Geometry check sheet. Reference: the model listing, model coordinates, mm. A direction names the side the tool comes from. Round coordinates to 2 decimals unless told otherwise and drop trailing zeros. Order: outer loops, then holes, each group sorted by start corner. A loop starts at its lowest first (then second) coordinate and runs counter-clockwise, first axis right, second up.
(1) Cross-section at B-B on x = 50. Enter the section's corners in (y, z) (3 decimals), and give its area (3 significant figures).
(2) Set-up check for faces 1 (the face through (-1, 42, -55)), 2 (the face through (-66.869, 8.351, -77.185)), 3 (the face through (64.545, 49, -44)): record each of +Z, -Z, +X, -X, +Y, -Y from which the full face is reachable in a straight line by a thin tool's end or side.
(3) Cross-section at C-C on y = 30. Enter the section's corners in (x, z) (3 decimals).
(4) Thickness scan on L1, parallel to Z at x = -39, y = 37 (3 decimals); L2, parallel to X at y = 35.5, z = -9.5 (3 decimals); L3, parallel to Y at x = -33.5, z = -15.5 (3 decimals). Record the ranges inside material, lowest first.
(5) Gauge pin test, flat ends, axial feed: P1, Ø1, axis at y = -34, z = -53.5, coming from the +X side; P2, Ø5, axis at y = 29, z = -65.5, coming from the +X side; P3, Ø6, axis at y = -37.5, z = -73.5, coming from the -X side; P4, Ø10.5, axis at x = -25.5, y = 41.5, coming from the -Z side. Record the tip position at first contact, or that the pin passes through.
(6) Draft check along Y on faces 4 (the face through (-1, 1, 0)), 5 (the face through (-1, 48.755, -28)), 6 (the face through (-1, 50, -27)). Enter one of: pulls with the +Y half, pulls with the -Y half, needs draft (parallel to the pull), parting line crosses it, or undercut.
(7) Cross-section at D-D on y = -15.5. Enter the section's corners in (x, z) (3 decimals), and give its area (3 significant figures).
(8) Cross-section at A-A on z = -29.5. Enter the section's corners in (x, y) (3 decimals), and give its area (3 significant figures).
from build123d import *

# Parameters (mm, degrees)
SKETCH1_W                      = 155
SKETCH1_H                      = 100
BASE_FLANGE2_DEPTH             = 1.245
EDGE_FLANGE3_STRIP_W           = 8.4
EDGE_FLANGE3_STRIP_H           = 1.245
EDGE_FLANGE3_STRIP_CUT_DEPTH   = 155
EDGE_FLANGE3_DEPTH             = 155
CUT_EXTRUDE2_START             = -1.245
CUT_EXTRUDE2_OUTLINE_W         = 10
CUT_EXTRUDE2_OUTLINE_H         = 102
CUT_EXTRUDE2_DEPTH             = 2.955
EDGE_FLANGE4_STRIP_W           = 8.4
EDGE_FLANGE4_STRIP_H           = 1.245
EDGE_FLANGE4_STRIP_CUT_DEPTH   = 97.045
EDGE_FLANGE4_STRIP_2_W         = 8.4
EDGE_FLANGE4_STRIP_2_H         = 1.245
EDGE_FLANGE4_STRIP_CUT_2_DEPTH = 97.045
EDGE_FLANGE4_DEPTH             = 97.045
EDGE_FLANGE4_BEND_DEPTH        = 97.045
EDGE_FLANGE5_STRIP_W           = 8.4
EDGE_FLANGE5_STRIP_H           = 1.245
EDGE_FLANGE5_STRIP_CUT_DEPTH   = 129.09
EDGE_FLANGE5_DEPTH             = 129.09
CUT_EXTRUDE3_DEPTH             = 192.224057064
EDGE_FLANGE6_STRIP_W           = 8.4
EDGE_FLANGE6_STRIP_H           = 1.245
EDGE_FLANGE6_STRIP_CUT_DEPTH   = 129.09
EDGE_FLANGE6_DEPTH             = 129.09
EDGE_FLANGE7_START             = -64.545
EDGE_FLANGE7_DEPTH             = 129.09
EDGE_FLANGE7_2_DEPTH           = 129.09


# Read off the part's stored shape, not the designer's step: Cut-Extrude2, Edge-Flange7
# Sheet-metal steps are written as plain solids
with BuildPart() as part:
    # Sketch1 → Base-Flange2 (new body)
    with BuildSketch(Plane.XY):
        Rectangle(SKETCH1_W, SKETCH1_H)
    extrude(amount=-BASE_FLANGE2_DEPTH)

    # Edge-Flange3 strip (across the edge) → Edge-Flange3 strip cut (cut)
    with BuildSketch(Plane(origin=(77.5, -50, -1.245), x_dir=(0, 1, 0), z_dir=(-1, 0, 0))):
        with Locations((-1.245, -0.6225)):
            Rectangle(EDGE_FLANGE3_STRIP_W, EDGE_FLANGE3_STRIP_H)
    extrude(amount=EDGE_FLANGE3_STRIP_CUT_DEPTH, mode=Mode.SUBTRACT)

    # Edge-Flange3 section (across the edge) → Edge-Flange3 (add)
    with BuildSketch(Plane(origin=(77.5, -50, -1.245), x_dir=(0, 1, 0), z_dir=(-1, 0, 0))):
        with BuildLine():
            Line((0, 1.71), (0, 112.955))
            Line((0, 112.955), (1.245, 112.955))
            Line((1.245, 112.955), (1.245, 1.71))
            ThreePointArc((1.245, 1.71), (1.745847404, 0.500847404), (2.955, 0))
            Line((2.955, 0), (2.955, -1.245))
            ThreePointArc((2.955, -1.245), (0.865499462, -0.379500538), (0, 1.71))
        make_face()
    extrude(amount=EDGE_FLANGE3_DEPTH)

    # Cut-Extrude2 outline → Cut-Extrude2 (cut)
    with BuildSketch(Plane(origin=(0, 0, -1.245), x_dir=(-1, 0, 0), z_dir=(0, 0, -1)).offset(CUT_EXTRUDE2_START)):
        with Locations((72.5, 0)):
            Rectangle(CUT_EXTRUDE2_OUTLINE_W, CUT_EXTRUDE2_OUTLINE_H)
        with Locations((-72.5, 0)):
            Rectangle(CUT_EXTRUDE2_OUTLINE_W, CUT_EXTRUDE2_OUTLINE_H)
    extrude(amount=CUT_EXTRUDE2_DEPTH, mode=Mode.SUBTRACT)

    # Edge-Flange4 strip (across the edge) → Edge-Flange4 strip cut (cut)
    with BuildSketch(Plane(origin=(67.5, 50, -1.245), x_dir=(-1, 0, 0), z_dir=(0, -1, 0))):
        with Locations((-1.245, -0.6225)):
            Rectangle(EDGE_FLANGE4_STRIP_W, EDGE_FLANGE4_STRIP_H)
    extrude(amount=EDGE_FLANGE4_STRIP_CUT_DEPTH, mode=Mode.SUBTRACT)

    # Edge-Flange4 strip 2 (across the edge) → Edge-Flange4 strip cut 2 (cut)
    with BuildSketch(Plane(origin=(-67.5, -47.045, -1.245), x_dir=(1, 0, 0), z_dir=(0, 1, 0))):
        with Locations((-1.245, -0.6225)):
            Rectangle(EDGE_FLANGE4_STRIP_2_W, EDGE_FLANGE4_STRIP_2_H)
    extrude(amount=EDGE_FLANGE4_STRIP_CUT_2_DEPTH, mode=Mode.SUBTRACT)

    # Edge-Flange4 section (across the edge) → Edge-Flange4 (add)
    with BuildSketch(Plane(origin=(67.5, 50, -1.245), x_dir=(-1, 0, 0), z_dir=(0, -1, 0))):
        with BuildLine():
            Line((0, 1.71), (0, 98.755))
            Line((0, 98.755), (1.245, 98.755))
            Line((1.245, 98.755), (1.245, 1.71))
            ThreePointArc((1.245, 1.71), (1.745847404, 0.500847404), (2.955, 0))
            Line((2.955, 0), (2.955, -1.245))
            ThreePointArc((2.955, -1.245), (0.865499462, -0.379500538), (0, 1.71))
        make_face()
    extrude(amount=EDGE_FLANGE4_DEPTH)

    # Edge-Flange4 section 2 (across the edge) → Edge-Flange4 bend (add)
    with BuildSketch(Plane(origin=(-67.5, -47.045, -1.245), x_dir=(1, 0, 0), z_dir=(0, 1, 0))):
        with BuildLine():
            Line((0, 1.71), (0, 98.755))
            Line((0, 98.755), (1.245, 98.755))
            Line((1.245, 98.755), (1.245, 1.71))
            ThreePointArc((1.245, 1.71), (1.745847404, 0.500847404), (2.955, 0))
            Line((2.955, 0), (2.955, -1.245))
            ThreePointArc((2.955, -1.245), (0.865499462, -0.379500538), (0, 1.71))
        make_face()
    extrude(amount=EDGE_FLANGE4_BEND_DEPTH)

    # Edge-Flange5 strip (across the edge) → Edge-Flange5 strip cut (cut)
    with BuildSketch(Plane(origin=(-64.545, 50, -1.245), x_dir=(0, -1, 0), z_dir=(1, 0, 0))):
        with Locations((-1.245, -0.6225)):
            Rectangle(EDGE_FLANGE5_STRIP_W, EDGE_FLANGE5_STRIP_H)
    extrude(amount=EDGE_FLANGE5_STRIP_CUT_DEPTH, mode=Mode.SUBTRACT)

    # Edge-Flange5 section (across the edge) → Edge-Flange5 (add)
    with BuildSketch(Plane(origin=(-64.545, 50, -1.245), x_dir=(0, -1, 0), z_dir=(1, 0, 0))):
        with BuildLine():
            Line((0, 1.71), (0, 53.755))
            Line((0, 53.755), (1.245, 53.755))
            Line((1.245, 53.755), (1.245, 1.71))
            ThreePointArc((1.245, 1.71), (1.745847404, 0.500847404), (2.955, 0))
            Line((2.955, 0), (2.955, -1.245))
            ThreePointArc((2.955, -1.245), (0.865499462, -0.379500538), (0, 1.71))
        make_face()
    extrude(amount=EDGE_FLANGE5_DEPTH)

    # Sketch26 → Cut-Extrude3 (cut, through all)
    with BuildSketch(Plane(origin=(67.5, 0, 0), x_dir=(0, 0, -1), z_dir=(1, 0, 0))):
        Polygon((55, 50), (55, 34.789940387), (100, -18.83897128), (100, 50), align=None)
    extrude(amount=-CUT_EXTRUDE3_DEPTH, mode=Mode.SUBTRACT)

    # Edge-Flange6 strip (across the edge) → Edge-Flange6 strip cut (cut)
    with BuildSketch(Plane(origin=(-64.545, 48.755, -55), x_dir=(0, 0, 1), z_dir=(1, 0, 0))):
        with Locations((-1.245, -0.6225)):
            Rectangle(EDGE_FLANGE6_STRIP_W, EDGE_FLANGE6_STRIP_H)
    extrude(amount=EDGE_FLANGE6_STRIP_CUT_DEPTH, mode=Mode.SUBTRACT)

    # Edge-Flange6 section (across the edge) → Edge-Flange6 (add)
    with BuildSketch(Plane(origin=(-64.545, 48.755, -55), x_dir=(0, 0, 1), z_dir=(1, 0, 0))):
        with BuildLine():
            Line((0, 1.71), (0, 13.965059613))
            Line((0, 13.965059613), (1.245, 13.965059613))
            Line((1.245, 13.965059613), (1.245, 1.71))
            ThreePointArc((1.245, 1.71), (1.745847404, 0.500847404), (2.955, 0))
            Line((2.955, 0), (2.955, -1.245))
            ThreePointArc((2.955, -1.245), (0.865499462, -0.379500538), (0, 1.71))
        make_face()
    extrude(amount=EDGE_FLANGE6_DEPTH)

    # Edge-Flange7 outline → Edge-Flange7 (cut)
    with BuildSketch(Plane.YZ.offset(EDGE_FLANGE7_START)):
        with BuildLine():
            Line((34.789940387, -55), (35.449768265, -54.446338671))
            ThreePointArc((35.449768265, -54.446338671), (36.338536128, -53.933208306), (37.349205652, -53.755))
            Line((37.349205652, -53.755), (34.789940387, -53.755))
            Line((34.789940387, -53.755), (34.789940387, -55))
        make_face()
    extrude(amount=EDGE_FLANGE7_DEPTH, mode=Mode.SUBTRACT)

    # Edge-Flange7 2 outline → Edge-Flange7 2 (add)
    with BuildSketch(Plane.YZ.offset(EDGE_FLANGE7_START)):
        with BuildLine():
            Line((37.349205652, -55), (34.789940387, -55))
            Line((34.789940387, -55), (-1.798735213, -85.701544201))
            Line((-1.798735213, -85.701544201), (-0.998464639, -86.655269533))
            Line((-0.998464639, -86.655269533), (36.250038839, -55.400064002))
            ThreePointArc((36.250038839, -55.400064002), (36.764351207, -55.103125618), (37.349205652, -55))
        make_face()
    extrude(amount=EDGE_FLANGE7_2_DEPTH)


solid = part.part
Found:
1. outline: (-50, -114.2) - (-48.755, -114.2) - (-48.755, -2.955) arc R1.71 cw to (-47.045, -1.245) - (47.045, -1.245) arc R1.71 cw to (48.755, -2.955) - (48.755, -52.045) arc R1.71 cw to (47.045, -53.755) - (37.349, -53.755) arc R2.955 ccw to (35.45, -54.446) - (-1.799, -85.702) - (-0.998, -86.655) - (36.25, -55.4) arc R1.71 cw to (37.349, -55) - (47.045, -55) arc R2.955 ccw to (50, -52.045) - (50, -2.955) arc R2.955 ccw to (47.045, 0) - (-47.045, 0) arc R2.955 ccw to (-50, -2.955) - close
1. area: 405 mm2
2. face 1: -Z, +X, -X, +Y
2. face 2: -Z, -X, +Y
2. face 3: -Z, +Y
3. outline: (-67.5, -59.019) - (-66.255, -59.019) - (-66.255, -2.955) arc R1.71 cw to (-64.545, -1.245) - (64.545, -1.245) arc R1.71 cw to (66.255, -2.955) - (66.255, -59.019) - (67.5, -59.019) - (67.5, -2.955) arc R2.955 ccw to (64.545, 0) - (-64.545, 0) arc R2.955 ccw to (-67.5, -2.955) - close; (-64.545, -60.644) - (64.545, -60.644) - (64.545, -59.019) - (-64.545, -59.019) - close
4. L1: z = -55.036 to -53.776, -1.245 to 0
4. L2: x = -67.5 to -66.255, 66.255 to 67.5
4. L3: y = -50 to -48.755, 48.755 to 50
5. P1: stops at x = 67.5
5. P2: passes through
5. P3: stops at x = -67.5
5. P4: stops at z = -55.4
6. face 4: needs draft
6. face 5: undercut
6. face 6: pulls with the +Y half
7. outline: (-67.5, -97.198) - (-66.255, -97.198) - (-66.255, -2.955) arc R1.71 cw to (-64.545, -1.245) - (64.545, -1.245) arc R1.71 cw to (66.255, -2.955) - (66.255, -97.198) - (67.5, -97.198) - (67.5, -2.955) arc R2.955 ccw to (64.545, 0) - (-64.545, 0) arc R2.955 ccw to (-67.5, -2.955) - close
7. area: 405 mm2
8. outline: (-77.5, -50) - (77.5, -50) - (77.5, -48.755) - (-77.5, -48.755) - close; (-67.5, -47.045) - (-66.255, -47.045) - (-66.255, 50) - (-67.5, 50) - close; (-64.545, 48.755) - (64.545, 48.755) - (64.545, 50) - (-64.545, 50) - close; (66.255, -47.045) - (67.5, -47.045) - (67.5, 50) - (66.255, 50) - close
8. area: 595 mm2
